Geometry: see drawing. Coordinates: mm, zero at the bounding-box minimum. Give positions to 0.01 mm unless a question says otherwise; leave off trailing zeros. Order: outer loops, then holes, each group sorted by start corner. A loop starts at its lowest first (then second) coordinate and runs counter-clockwise, first axis right, second up. Notation, with made-up numbers: (1.25, 36) -> (37.25, 36) arc R29 ccw to (37.25, 64) -> close; hole circle Ø11 at (86.25, -27.5). An arc over 180 degrees is marked (long way). Use one line per item in the form item = value. Start each with the question number.
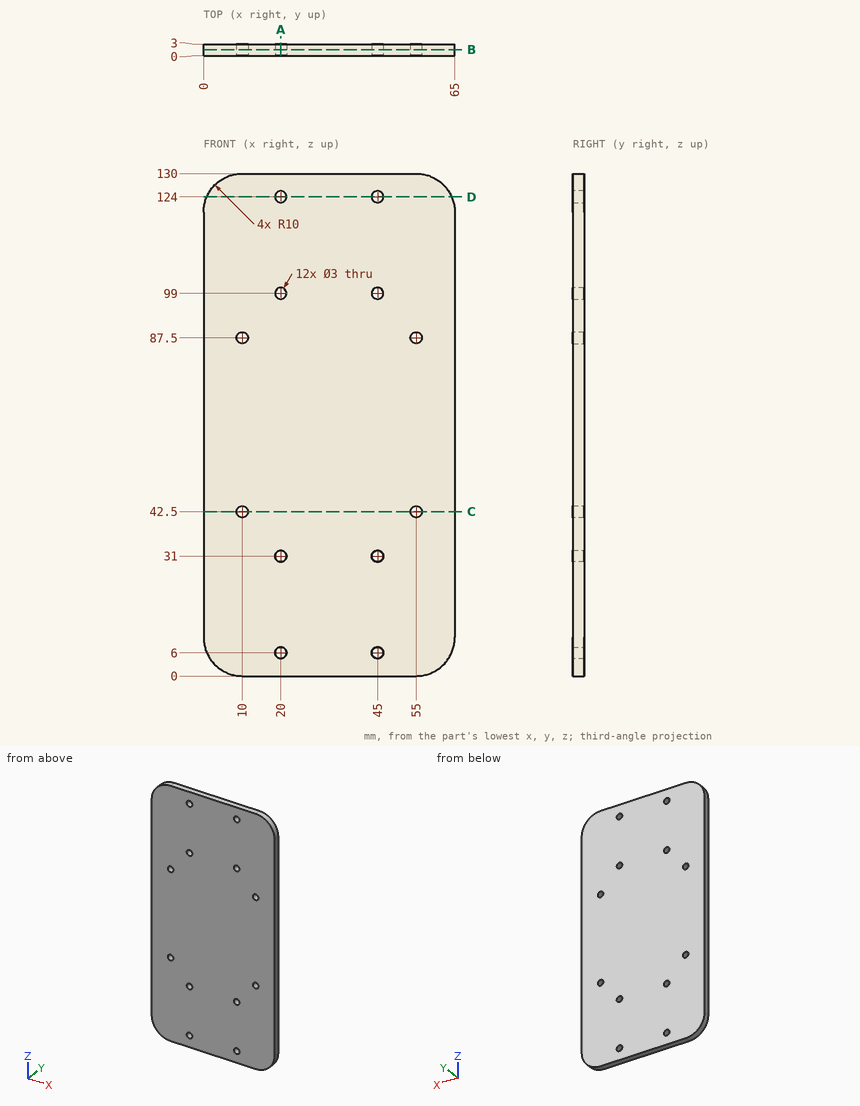
1) Cut plane D-D, the plane z = 124. Return the cut outline in (x, y), plus the area to 3 significant figures.
2) Cut plane B-B, the plane y = 1.55. Count the separate pieces of the cut face and the enclosed holes in it, plus the area to 3 significant figures.
3) Pin query (flat end, axial travel): pin 1 (1.8 mm diameter, centred on x = 55, z = 87.5, fed in from +Y); pin 2 (5 mm diameter, centred on x = 10, z = 87.5, fed in from +Y). Return the tip coordinate at first contact, or that it passes through.
4) Cut plane A-A, the plane x = 20. Return the cut outline in (y, z).
5) Cut plane C-C, the plane z = 42.5. Return the cut outline in (x, y).
6) Material intervals for probe 1 along X at (y, z) = (1.95, 124); probe 2 along Z at (x, y) = (61.5, 1.8); probe 3 along X at (y, z) = (1.8, 8), sorted ascending.
Output values:
q1.outline = (0.83, 0) -> (18.5, 0) -> (18.5, 3) -> (0.83, 3) -> close; (21.5, 0) -> (43.5, 0) -> (43.5, 3) -> (21.5, 3) -> close; (46.5, 0) -> (64.17, 0) -> (64.17, 3) -> (46.5, 3) -> close
q1.area = 172 mm^2
q2.separate_pieces = 1
q2.enclosed_holes = 12
q2.area = 8,280 mm^2
q3.pin_1 = through
q3.pin_2 = 3
q4.outline = (0, 0) -> (3, 0) -> (3, 4.5) -> (0, 4.5) -> close; (0, 7.5) -> (3, 7.5) -> (3, 29.5) -> (0, 29.5) -> close; (0, 32.5) -> (3, 32.5) -> (3, 97.5) -> (0, 97.5) -> close; (0, 100.5) -> (3, 100.5) -> (3, 122.5) -> (0, 122.5) -> close; (0, 125.5) -> (3, 125.5) -> (3, 130) -> (0, 130) -> close
q5.outline = (0, 0) -> (8.5, 0) -> (8.5, 3) -> (0, 3) -> close; (11.5, 0) -> (53.5, 0) -> (53.5, 3) -> (11.5, 3) -> close; (56.5, 0) -> (65, 0) -> (65, 3) -> (56.5, 3) -> close
q6.probe_1 = 0.83 to 18.5, 21.5 to 43.5, 46.5 to 64.17
q6.probe_2 = 2.4 to 127.6
q6.probe_3 = 0.2 to 64.8
